CAD build for the part. Positions are in the model's coordinates, mm. Face numbers are marked on the shaded views. A direction names the side the tool comes from. Coordinates: 2 decimals unless noted, no trailing zeros. Loops run counter-clockwise (first coordinate to the right, second up) from the corner with the lowest first, then second, coordinate; pieces in that order, holes last. Notation, with made-up numbers: (5, 5.5) -> (12, 5.5) arc R18 ccw to (12, 14.5) -> close; hole circle Ø6 at (17, -37.5). An arc over 180 degrees is marked (long way). Write each question's results on one line, items separated by ' | '.
from build123d import *

# Parameters (mm, degrees)
SKETCH1_W           = 30
SKETCH1_H           = 60
BOSS_EXTRUDE1_DEPTH = 12
SKETCH2_R           = 3
BOSS_EXTRUDE2_DEPTH = 60
SKETCH3_W           = 12
SKETCH3_H           = 7.5
CUT_EXTRUDE1_DEPTH  = 69.14690015
LPATTERN1_COUNT     = 4
LPATTERN1_PITCH     = 15
SKETCH4_R           = 1.75
CUT_EXTRUDE2_DEPTH  = 69.14690015
SKETCH5_R           = 5
CUT_EXTRUDE3_DEPTH  = 3
LPATTERN2_COUNT     = 2
LPATTERN2_PITCH     = 9


with BuildPart() as part:
    # Sketch1 → Boss-Extrude1 (new body)
    with BuildSketch(Plane(origin=(0, 0, 0), x_dir=(1, 0, 0), z_dir=(0, 1, 0))):
        with Locations((-15, 30)):
            Rectangle(SKETCH1_W, SKETCH1_H)
    extrude(amount=BOSS_EXTRUDE1_DEPTH)

    # Sketch2 → Boss-Extrude2 (add)
    with BuildSketch(Plane.XY):
        with BuildLine():
            Line((0, 6), (0, 0))
            Line((0, 0), (6, 0))
            ThreePointArc((6, 0), (12, 6), (6, 12))
            Line((6, 12), (0, 12))
            Line((0, 12), (0, 6))
        make_face()
        with Locations((6, 6)):
            Circle(SKETCH2_R, mode=Mode.SUBTRACT)
    extrude(amount=-BOSS_EXTRUDE2_DEPTH)

    # Sketch3 → Cut-Extrude1 (cut, through all)
    with BuildSketch(Plane(origin=(0, 12, 0), x_dir=(1, 0, 0), z_dir=(0, 1, 0))):
        with Locations((6, 48.75)):
            Rectangle(SKETCH3_W, SKETCH3_H)
    cut_extrude1 = extrude(amount=-CUT_EXTRUDE1_DEPTH, mode=Mode.SUBTRACT)

    # LPattern1: Cut-Extrude1 ×4
    with Locations(*[(0, 0, i * LPATTERN1_PITCH) for i in range(1, LPATTERN1_COUNT)]):
        add(cut_extrude1, mode=Mode.SUBTRACT)

    # Sketch4 → Cut-Extrude2 (cut, through all)
    with BuildSketch(Plane(origin=(0, 12, 0), x_dir=(1, 0, 0), z_dir=(0, 1, 0))):
        with Locations(Location((-15, 45, 0), (0, 0, 270))):
            Circle(SKETCH4_R)
        with Locations(Location((-15, 15, 0), (0, 0, 270))):
            Circle(SKETCH4_R)
    extrude(amount=-CUT_EXTRUDE2_DEPTH, mode=Mode.SUBTRACT)

    # Sketch5 → Cut-Extrude3 (cut)
    with BuildSketch(Plane(origin=(0, 12, 0), x_dir=(1, 0, 0), z_dir=(0, 1, 0))):
        with Locations(Location((-15, 45, 0), (0, 0, 270))):
            Circle(SKETCH5_R)
        with Locations(Location((-15, 15, 0), (0, 0, 270))):
            Circle(SKETCH5_R)
    cut_extrude3 = extrude(amount=-CUT_EXTRUDE3_DEPTH, mode=Mode.SUBTRACT)

    # LPattern2: Cut-Extrude3 ×2
    with Locations(*[(0, -i * LPATTERN2_PITCH, 0) for i in range(1, LPATTERN2_COUNT)]):
        add(cut_extrude3, mode=Mode.SUBTRACT)


solid = part.part
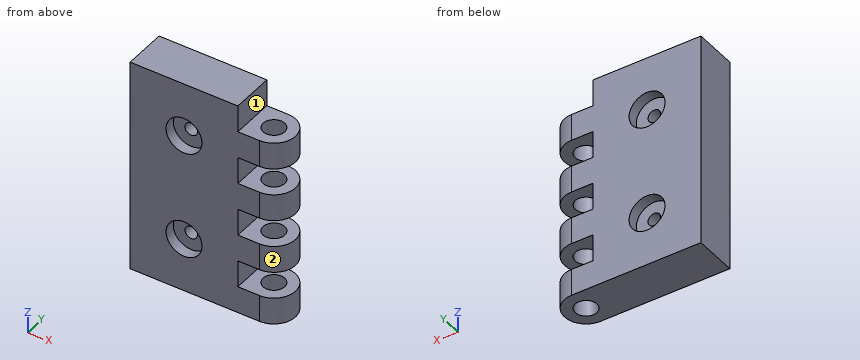
1) Drill centre lines: L1, parallel to Y at x = 6, z = -40; L2, parallel to Z at x = -15.5, y = 4.75; L3, parallel to Z at x = -13, y = 2. Where is each one in solid material? Low to high. Write a range as from..to.
Outcome:
L1: y = 0..3, 9..12 | L2: z = -60..-46.68, -43.32..-16.68, -13.32..0 | L3: z = -60..-49.58, -40.42..-19.58, -10.42..0
2) Slice it at A-A (x = -15). Write the cut outline in (y, z), then the cut area to 3 significant figures.
Outcome:
outline: (0, -60) -> (12, -60) -> (12, -50) -> (9, -50) -> (9, -46.75) -> (3, -46.75) -> (3, -50) -> (0, -50) -> close; (0, -40) -> (3, -40) -> (3, -43.25) -> (9, -43.25) -> (9, -40) -> (12, -40) -> (12, -20) -> (9, -20) -> (9, -16.75) -> (3, -16.75) -> (3, -20) -> (0, -20) -> close; (0, -10) -> (3, -10) -> (3, -13.25) -> (9, -13.25) -> (9, -10) -> (12, -10) -> (12, 0) -> (0, 0) -> close | area: 558 mm^2
3) Pin check, flat tips, straight feed: pin 1 (4 mm diameter, centred on x = -15, z = -45, fed in from -Y); pin 2 (3.5 mm diameter, centred on x = 6, y = 4, fed in from +Z). Stop position of each tip, or through.
Outcome:
pin 1: stops at y = 3 | pin 2: stops at z = -7.5
4) Slice it at C-C (y = 4.75). Count the separate pieces of the cut face and the enclosed holes in it, then the cut area to 3 significant figures.
Outcome:
separate pieces: 5 | enclosed holes: 2 | area: 1,970 mm^2
5) Slice it at D-D (z = -11.5). Write the cut outline in (x, y).
Outcome:
outline: (-30, 0) -> (-18.57, 0) -> (-18.57, 3) -> (-11.43, 3) -> (-11.43, 0) -> (6, 0) arc R6 ccw to (6, 12) -> (-11.43, 12) -> (-11.43, 9) -> (-18.57, 9) -> (-18.57, 12) -> (-30, 12) -> close; hole circle Ø6 at (6, 6)
6) Which spindle directions (+Z, -Z, +X, -X, +Y, -Y) get a long thin tool onto all of the face, cutting with end or side? Do the marked faces 1 and 2. Say none if no direction does.
Outcome:
face 1: +Z, +X, +Y, -Y | face 2: +Z, -Z, +X
7) Slice it at B-B (x = 1). Write the cut outline in (y, z).
Outcome:
outline: (0, -60) -> (12, -60) -> (12, -52.5) -> (0, -52.5) -> close; (0, -45) -> (12, -45) -> (12, -37.5) -> (0, -37.5) -> close; (0, -30) -> (12, -30) -> (12, -22.5) -> (0, -22.5) -> close; (0, -15) -> (12, -15) -> (12, -7.5) -> (0, -7.5) -> close
